from build123d import *

# Parameters (mm, degrees)
BOSS_EXTRUDE1_DEPTH = 23.6474
CUT_EXTRUDE1_START  = -15.748
CUT_EXTRUDE1_DEPTH  = 15.748
SKETCH3_R           = 3.175
BOSS_EXTRUDE2_DEPTH = 55.88
BOSS_EXTRUDE3_DEPTH = 11.43
CHAMFER1_SIZE       = 1.778


with BuildPart() as part:
    # Sketch1 → Boss-Extrude1 (new body)
    with BuildSketch(Plane.XY):
        with BuildLine():
            Line((0.695350686, 9.200310447), (63.61372159, 4.445))
            ThreePointArc((63.61372159, 4.445), (67.73545, 0), (63.61372159, -4.445))
            Line((63.61372159, -4.445), (0.695350686, -9.200310447))
            ThreePointArc((0.695350686, -9.200310447), (-9.22655, 0), (0.695350686, 9.200310447))
        make_face()
    extrude(amount=-BOSS_EXTRUDE1_DEPTH)

    # Sketch2 → Cut-Extrude1 (cut)
    with BuildSketch(Plane(origin=(0, 0, -23.6474), x_dir=(-1, 0, 0), z_dir=(0, 0, -1)).offset(CUT_EXTRUDE1_START)):
        with BuildLine():
            Line((-0.695350686, 9.200310447), (-63.61372159, 4.445))
            ThreePointArc((-63.61372159, 4.445), (-67.73545, 0), (-63.61372159, -4.445))
            Line((-63.61372159, -4.445), (-0.695350686, -9.200310447))
            ThreePointArc((-0.695350686, -9.200310447), (9.22655, 0), (-0.695350686, 9.200310447))
        make_face()
        with BuildLine():
            Line((-0.653237224, 8.643099629), (-63.571608128, 3.887789181))
            ThreePointArc((-63.571608128, 3.887789181), (-67.17665, 0), (-63.571608128, -3.887789181))
            Line((-63.571608128, -3.887789181), (-0.653237224, -8.643099629))
            ThreePointArc((-0.653237224, -8.643099629), (8.66775, 0), (-0.653237224, 8.643099629))
        make_face(mode=Mode.SUBTRACT)
    extrude(amount=CUT_EXTRUDE1_DEPTH, mode=Mode.SUBTRACT)

    # Sketch3 → Boss-Extrude2 (add)
    with BuildSketch(Plane.XY):
        Circle(SKETCH3_R)
    extrude(amount=BOSS_EXTRUDE2_DEPTH)

    # Sketch4 → Boss-Extrude3 (add)
    with BuildSketch(Plane(origin=(0, 0, -7.8994), x_dir=(-1, 0, 0), z_dir=(0, 0, -1))):
        with BuildLine():
            Line((-0.933674597, 12.353617125), (-63.852045501, 7.598306678))
            ThreePointArc((-63.852045501, 7.598306678), (-70.89775, 0), (-63.852045501, -7.598306678))
            Line((-63.852045501, -7.598306678), (-0.933674597, -12.353617125))
            ThreePointArc((-0.933674597, -12.353617125), (12.38885, 0), (-0.933674597, 12.353617125))
        make_face()
        with BuildLine():
            Line((-0.653237224, 8.643099629), (-63.571608128, 3.887789181))
            ThreePointArc((-63.571608128, 3.887789181), (-67.17665, 0), (-63.571608128, -3.887789181))
            Line((-63.571608128, -3.887789181), (-0.653237224, -8.643099629))
            ThreePointArc((-0.653237224, -8.643099629), (8.66775, 0), (-0.653237224, 8.643099629))
        make_face(mode=Mode.SUBTRACT)
    extrude(amount=BOSS_EXTRUDE3_DEPTH)

    # Chamfer1
    chamfer1_edges = [part.edges().sort_by_distance(p)[0] for p in [
        (-3.175, 0, 55.88),
    ]]
    chamfer(chamfer1_edges, length=CHAMFER1_SIZE)


solid = part.part
Input: part model. Units: mm. Frame: model coordinates. A direction names the side the tool comes from. Give positions to 0.01 mm unless a question says otherwise; leave off trailing zeros. Write each loop counter-clockwise with the first axis right and the second up, starting at its lowest first coordinate (ties: lowest second). Pieces come first, ordered by that corner, then holes. Notation, with made-up numbers: (-1, 43) -> (52, 43) arc R12 cw to (52, 59) -> close; hole circle Ø3 at (50, 76). An arc over 180 degrees is marked (long way). Use one line per item in the form item = value. Start each with the question number.
1) Section query A-A on y = 0. Return the cut outline in (x, z) (3 decimals), then the cut area to 3 significant figures.
2) Set-up query: faces 1 (the flat face through (31.67, 6.3, -21.46)), 2 (the flat face through (32.553, -6.232, -21.458)), 3 (the flat face through (31.714, 6.856, -3.894)), 4 (the cylindrical face through (67.176, 0.082, -21.458)). Return all of +Z, -Z, +X, -X, +Y, -Y with unobstructed straight access to the full face (end or side cutting, diameter ignored); none if empty.
3) Pin query (flat end, axial travel): pin 1 (9 mm diameter, centred on x = 47, y = -3, fed in from +Z); pin 2 (12 mm diameter, centred on y = -5.5, z = 33, fed in from +X) (3 decimals); pin 3 (3 mm diameter, centred on x = 7.5, z = -14.5, fed in from -Y). Return the tip coordinate at first contact, or that it passes through.
4) Section query C-C on x = 41. Return the cut outline in (y, z), then the cut area to 3 significant figures.
5) Ray query, probe 1 along Z at (x, y) = (24.5, 4.25); probe 2 along Z at (x, y) = (14, 7.75); probe 3 along X at (y, z) = (-0.5, 5). Return the intervals inside material, ascending. Write a range as from..to.
6) Section query B-B on z = 38.5. Return the cut outline in (x, y) (3 decimals), then the cut area to 3 significant figures.
7) Section query D-D on x = 12.5. Return the cut outline in (y, z), then the cut area to 3 significant figures.
Outcome:
q1.outline = (-12.389, -19.329) -> (-8.668, -19.329) -> (-8.668, -23.647) -> (67.177, -23.647) -> (67.177, -19.329) -> (70.898, -19.329) -> (70.898, -7.899) -> (67.735, -7.899) -> (67.735, 0) -> (3.175, 0) -> (3.175, 54.102) -> (1.397, 55.88) -> (-1.397, 55.88) -> (-3.175, 54.102) -> (-3.175, 0) -> (-9.227, 0) -> (-9.227, -7.899) -> (-12.389, -7.899) -> close
q1.area = 2,240 mm^2
q2.face_1 = -Z, +X, +Y
q2.face_2 = -Z, +X, -Y
q2.face_3 = +Z, +X, +Y
q2.face_4 = -Z, +X
q3.pin_1 = 0
q3.pin_2 = 3.175
q3.pin_3 = -11.97
q4.outline = (-9.33, -19.33) -> (-5.59, -19.33) -> (-5.59, -23.65) -> (5.59, -23.65) -> (5.59, -19.33) -> (9.33, -19.33) -> (9.33, -7.9) -> (6.15, -7.9) -> (6.15, 0) -> (-6.15, 0) -> (-6.15, -7.9) -> (-9.33, -7.9) -> close
q4.area = 359 mm^2
q5.probe_1 = -23.65..0
q5.probe_2 = -19.33..0
q5.probe_3 = -3.14..3.14
q6.outline = circle Ø6.35 at (0, 0)
q6.area = 31.7 mm^2
q7.outline = (-11.48, -19.33) -> (-7.75, -19.33) -> (-7.75, -23.65) -> (7.75, -23.65) -> (7.75, -19.33) -> (11.48, -19.33) -> (11.48, -7.9) -> (8.31, -7.9) -> (8.31, 0) -> (-8.31, 0) -> (-8.31, -7.9) -> (-11.48, -7.9) -> close
q7.area = 461 mm^2
